```python
from build123d import *

# Parameters (mm, degrees)
SKETCH_W     = 12
SKETCH_H     = 14
SKETCH_R     = 2.5
PAD_DEPTH    = 3
SKETCH001_W  = 2
SKETCH001_H  = 14
PAD001_DEPTH = 16
SKETCH002_W  = 14
SKETCH002_H  = 3
PAD008_DEPTH = 10
SKETCH004_W  = 14
SKETCH004_H  = 3
PAD004_DEPTH = 8
SKETCH003_W  = 34
SKETCH003_H  = 3
PAD009_DEPTH = 8
SKETCH006_R  = 2
POCKET_DEPTH = 19.001
PAD005_DEPTH = 3
SKETCH008_W  = 19
SKETCH008_H  = 19
PAD010_DEPTH = 3
SKETCH009_W  = 2
SKETCH009_H  = 19
PAD011_DEPTH = 3
CHAMFER_SIZE = 1.5
FILLET_R     = 1
FILLET001_R  = 1
FILLET002_R  = 1
FILLET003_R  = 0.5
FILLET004_R  = 1


with BuildPart() as part:
    # Sketch → Pad (new body)
    with BuildSketch(Plane.XY):
        with Locations((-1, 0)):
            Rectangle(SKETCH_W, SKETCH_H)
        Circle(SKETCH_R, mode=Mode.SUBTRACT)
    extrude(amount=PAD_DEPTH)

    # Sketch001 (on Face7 of Pad) → Pad001 (join)
    with BuildSketch(Plane.XY.offset(3)):
        with Locations((-6, 0)):
            Rectangle(SKETCH001_W, SKETCH001_H)
    extrude(amount=PAD001_DEPTH)

    # Sketch002 (on Face10 of Pad001) → Pad008 (join)
    with BuildSketch(Plane.YZ.offset(-5)):
        with Locations((0, 17.5)):
            Rectangle(SKETCH002_W, SKETCH002_H)
    extrude(amount=PAD008_DEPTH)

    # Sketch004 → Pad004 (join)
    with BuildSketch(Plane(origin=(5, 0, 0), x_dir=(0, -1, 0), z_dir=(-1, 0, 0))):
        with Locations((0, 1.5)):
            Rectangle(SKETCH004_W, SKETCH004_H)
    extrude(amount=-PAD004_DEPTH)

    # Sketch003 → Pad009 (join)
    with BuildSketch(Plane(origin=(5, 0, 0), x_dir=(0, -1, 0), z_dir=(-1, 0, 0))):
        with Locations((-10, 17.5)):
            Rectangle(SKETCH003_W, SKETCH003_H)
    extrude(amount=-PAD009_DEPTH)

    # Sketch006 → Pocket (cut, through all)
    with BuildSketch(Plane.XY.offset(19)):
        with Locations((9, 22)):
            Circle(SKETCH006_R)
        with Locations((9, 12)):
            Circle(SKETCH006_R)
    extrude(amount=-POCKET_DEPTH, mode=Mode.SUBTRACT)

    # Sketch007 (on Face26 of Pocket) → Pad005 (join)
    with BuildSketch(Plane.YZ.offset(13)):
        Polygon((27, 19), (-7, 19), (-7, 0), (7, 0), (27, 16), align=None)
    extrude(amount=PAD005_DEPTH)

    # Sketch008 (on Face19 of Pad005) → Pad010 (join)
    with BuildSketch(Plane.XZ.offset(7)):
        with Locations((6.5, 9.5)):
            Rectangle(SKETCH008_W, SKETCH008_H)
    extrude(amount=PAD010_DEPTH)

    # Sketch009 (on Face14 of Pad010) → Pad011 (join)
    with BuildSketch(Plane.YZ.offset(-5)):
        with Locations((-6, 9.5)):
            Rectangle(SKETCH009_W, SKETCH009_H)
    extrude(amount=PAD011_DEPTH)

    # Chamfer
    chamfer_edges = [part.edges().sort_by_distance(p)[0] for p in [
        (-2, -5, 9.5),
    ]]
    chamfer(chamfer_edges, length=CHAMFER_SIZE)

    # Fillet
    fillet_edges = [part.edges().sort_by_distance(p)[0] for p in [
        (16, 0, 0),
    ]]
    fillet(fillet_edges, radius=FILLET_R)

    # Fillet001
    fillet001_edges = [part.edges().sort_by_distance(p)[0] for p in [
        (-7, 0, 0),
    ]]
    fillet(fillet001_edges, radius=FILLET001_R)

    # Fillet002
    fillet002_edges = [part.edges().sort_by_distance(p)[0] for p in [
        (5, 27, 17.5),
        (16, 27, 17.5),
    ]]
    fillet(fillet002_edges, radius=FILLET002_R)

    # Fillet003
    fillet003_edges = [part.edges().sort_by_distance(p)[0] for p in [
        (16, 9.5, 19),
        (5, 16.5, 19),
    ]]
    fillet(fillet003_edges, radius=FILLET003_R)

    # Fillet004
    fillet004_edges = [part.edges().sort_by_distance(p)[0] for p in [
        (-7, 0, 19),
    ]]
    fillet(fillet004_edges, radius=FILLET004_R)


solid = part.part
```
For this review, take the finished solid that the model builds, in its own axes (mm). A direction names the side the tool comes from. Coordinates: 2 decimals unless noted, no trailing zeros. Write each loop counter-clockwise with the first axis right and the second up, starting at its lowest first coordinate (ties: lowest second). Pieces come first, ordered by that corner, then holes. Notation, with made-up numbers: (-5, 53.25) - (25, 53.25) arc R27 ccw to (25, 91.25) - close; hole circle Ø4 at (-10.5, 37.5). An arc over 180 degrees is marked (long way). Put each result on its own line as item: value.
1. Add section D-D, the plane y = 17.5. Give the boundary of the cut face in (x, z).
Values found:
outline: (5, 16) - (13, 16) - (13, 8.4) - (16, 8.4) - (16, 18.5) arc R0.5 ccw to (15.5, 19) - (5.5, 19) arc R0.5 ccw to (5, 18.5) - close
2. For pin 1 (6 mm diameter, centred on x = 5, z = 16.5, fed in from +Y); pin 2 (9.5 mm diameter, centred on x = 4, z = 8, fed in from +Y); pin 3 (4 mm diameter, centred on y = 18, z = 7, fed in from -X); pin 4 (9 mm diameter, centred on x = 4, y = 15.5, fed in from -Z), all flat-tipped, find the tip position at first contact; note any pin that passes through.
Values found:
pin 1: y = 27
pin 2: y = -7
pin 3: x = 13
pin 4: z = 16
3. Machinability: for faces 1 (the flat face through (-5, -7, 10)), 2 (the flat face through (6, 6, 16)), 3 (the flat face through (6, -10, 10)), 4 (the cylindrical face through (-0.54, -2.44, 1.48)), which of the approach directions +Z, -Z, +X, -X, +Y, -Y give a long, thin tool a straight path to every point of the face, cutting with its end or side? Answer none if there is none.
Values found:
face 1: +Z, -Z, -X, -Y
face 2: +Y
face 3: +Z, -Z, +X, -X, -Y
face 4: -Z
4. Add section C-C, the plane x = 0. Give the boundary of the cut face in (y, z).
Values found:
outline: (-10, 0) - (-2.5, 0) - (-2.5, 3) - (-7, 3) - (-7, 16) - (7, 16) - (7, 19) - (-10, 19) - close; (2.5, 0) - (7, 0) - (7, 3) - (2.5, 3) - close
5. Add section A-A, the plane x = 9. Give the boundary of the cut face in (y, z), then the cut area to 3 significant figures.
Values found:
outline: (-10, 0) - (7, 0) - (7, 3) - (-7, 3) - (-7, 16) - (10, 16) - (10, 19) - (-10, 19) - close; (14, 16) - (20, 16) - (20, 19) - (14, 19) - close; (24, 16) - (27, 16) - (27, 18.5) arc R0.5 ccw to (26.5, 19) - (24, 19) - close
area: 177 mm²
6. Wall thickness on probe 1 along Y at (x, z) = (9, 18.25); probe 2 along Z at (x, y) = (12.5, -2); probe 3 along X at (y, z) = (3, 7.5): over which ranges is each line inside the solid? List them lowest first.
Values found:
probe 1: -10 to 10, 14 to 20, 24 to 27
probe 2: 0 to 3, 16 to 19
probe 3: -7 to -5, 13 to 16
7. Add section B-B, the plane y = 12. Give the boundary of the cut face in (x, z).
Values found:
outline: (5, 16) - (7, 16) - (7, 19) - (5.5, 19) arc R0.5 ccw to (5, 18.5) - close; (11, 16) - (13, 16) - (13, 4) - (16, 4) - (16, 18.5) arc R0.5 ccw to (15.5, 19) - (11, 19) - close
8. Mouldability with a two-part tool opening along Y and no side actions: class faces 5 (the flat face through (-7, 0, 9)), 6 (the cylindrical face through (15.715, 26.699, 17.24)), 7 (the cylindrical face through (9, 14, 18)) as released by +Y, released by -Y, zero draft, split by the parting line, or undercut.
Values found:
face 5: zero draft
face 6: released by +Y
face 7: undercut
